Here's how the part is built. I have some questions about the finished solid (model axes, mm). A direction names the side the tool comes from. Round coordinates to 2 decimals unless told otherwise and drop trailing zeros. Loops run counter-clockwise (first coordinate to the right, second up) from the corner with the lowest first, then second, coordinate; pieces in that order, holes last. Notation, with made-up numbers: (49.5, 80) -> (61.5, 80) arc R17 cw to (61.5, 95) -> close; hole circle Ø6 at (71, 24). An arc over 180 degrees is marked (long way). Use one line per item in the form item = value. Start each with the question number.
Item 1: If I drill on L1, parallel to X at y = 0.25, z = 3.5; L2, parallel to Y at x = 4, z = 0; L3, parallel to X at y = 0.5, z = 1.5, over which ranges is the centre line in solid material (lowest first)? Write a range as [from, to].
Item 2: Thinking about a two-plate mould opening in Z: for faces 4 (the face through (0, -1, -2)), 5 (the face through (11, -3, 0)), 6 (the face through (0.99, 0.99, 1.74)), which applies, released by +Z, released by -Z, zero draft, split by the parting line, or undercut?
Item 3: I'm going to push flat-ended pins straight in: pin 1 Ø1.5 at (x, z) = (7.5, 1.5) entering from +Y; pin 2 Ø3 at (y, z) = (-0.5, -3.5) entering from +X; pin 3 Ø1.5 at (x, y) = (11.5, 0.5) entering from -Z. Where does each tip first touch, or does it pass through?
Item 4: If we section it at B-B (x = 10.75): Write out the boundary of the cut face in (y, z).
Item 5: For faces 1 (the face through (1, 2, 0)), 2 (the face through (3.5, 2, 3)), 3 (the face through (19.5, 0, 0)), which set-ups out of +Z, -Z, +X, -X, +Y, -Y let a thin tool reach every point of the face, with its end or its side?
Item 6: If we section it at A-A (z = 0): Write out the boundary of the cut face in (x, y), then the cut area to 3 significant figures.
```python
from build123d import *

# Parameters (mm, degrees)
CUT_EXTRUDE_1_DEPTH = 2
FILLET_1_R          = 0.3
CHAMFER_1_SIZE      = 1


with BuildPart() as part:
    # Эскиз1 → Повернуть1 (revolve)
    with BuildSketch(Plane.XY):
        with BuildLine():
            Line((0, 0), (0, 4))
            ThreePointArc((0, 4), (1.41886117, 4.74341649), (3, 5))
            Line((3, 5), (3.5, 5))
            Line((3.5, 5), (3.5, 3))
            Line((3.5, 3), (19.5, 3))
            Line((19.5, 3), (19.5, 0))
            Line((19.5, 0), (0, 0))
        make_face()
    revolve(axis=Axis((19.5, 0, 0), (-1, 0, 0)))

    # Эскиз2 → Вырез-Вытянуть1 (cut)
    with BuildSketch(Plane.ZY):
        Polygon((1.154700538, 2), (-1.154700538, 2), (-2.309401077, 0), (-1.154700538, -2), (1.154700538, -2), (2.309401077, 0), align=None)
    extrude(amount=-CUT_EXTRUDE_1_DEPTH, mode=Mode.SUBTRACT)

    # Скругление1
    fillet_1_edges = [part.edges().sort_by_distance(p)[0] for p in [
        (3.5, -3, 0),
        (3.5, -5, 0),
    ]]
    fillet(fillet_1_edges, radius=FILLET_1_R)

    # Фаска1
    chamfer_1_edges = [part.edges().sort_by_distance(p)[0] for p in [
        (19.5, -3, 0),
    ]]
    chamfer(chamfer_1_edges, length=CHAMFER_1_SIZE)


solid = part.part
```
Values found:
q1.L1 = [0, 3.5]
q1.L2 = [-3, 3]
q1.L3 = [2, 19.5]
q2.face_4 = zero draft
q2.face_5 = split by the parting line
q2.face_6 = undercut
q3.pin_1 = 2.9
q3.pin_2 = 19.46
q3.pin_3 = -3
q4.outline = circle Ø6 at (0, 0)
q5.face_1 = -X
q5.face_2 = +X
q5.face_3 = +Z, -Z, +X, +Y, -Y
q6.outline = (0, -4) arc R5 ccw to (3, -5) -> (3.2, -5) arc R0.3 ccw to (3.5, -4.7) -> (3.5, -3.3) arc R0.3 cw to (3.8, -3) -> (18.5, -3) -> (19.5, -2) -> (19.5, 2) -> (18.5, 3) -> (3.8, 3) arc R0.3 cw to (3.5, 3.3) -> (3.5, 4.7) arc R0.3 ccw to (3.2, 5) -> (3, 5) arc R5 ccw to (0, 4) -> (0, 2) -> (2, 2) -> (2, -2) -> (0, -2) -> close
q6.area = 120 mm2
